Can you work these out from the model? Positions are in its coordinate system, mm. A direction names the side the tool comes from. Give positions to 0.01 mm unless a question says otherwise; leave off trailing zeros. Loops run counter-clockwise (first coordinate to the right, second up) from the corner with the lowest first, then second, coordinate; pieces in that order, holes last. Notation, with made-up numbers: M 72.25,69 L 92.25,69 A23 cw 92.25,91 Z; hole C -3.75,-29.5 d2. An arc over 180 degrees is marked long. Put each result on its own line as item: value. Start each with the question number.
1) Imagine slicing it at C-C (z = -20). Write out the boundary of the cut face in (x, y).
2) If we mould it in two halves opening along X, with no side actions, what happens to faces 1 (the flat face through (35, 0, -15)), 2 (the cylindrical face through (0.676, 0.088, -27.854)), 3 (the flat face through (30, 1, 0)), 4 (the cylindrical face through (-26.241, 2.685, 2.465))? For each: +X half, -X half, draft (parallel to the pull), parting line (faces both ways), or undercut.
3) Imagine slicing it at D-D (y = 3.5). Write out the boundary of the cut face in (x, z), then the cut area to 3 significant figures.
4) Please list where these lines run through material, in increasing order: line 1 along Z through (x, y) = (23.75, 1.5); line 2 along X through (y, z) = (-1.75, -25); line 3 along X through (y, z) = (-0.75, -18). Write a range as from..to.
5) Imagine slicing it at A-A (x = 23.75). Write out the boundary of the cut face in (y, z), then the cut area to 3 significant figures.
6) For P1, Ø6, axis at x = 23.75, z = -5.76, coming from the +Y side, with a flat end and sliding along its axis, tell me the tip position at first contact or that it passes through.
7) For faces 5 (the cylindrical face through (-26.241, 2.685, -32.535)), 6 (the cylindrical face through (-25.987, 1.476, -25.618)), which set-ups out of +Z, -Z, +X, -X, +Y, -Y let a thin tool reach every point of the face, with its end or its side?
8) Imagine slicing it at B-B (y = -3.75). State how many separate pieces and enclosed holes the cut face has, then the cut area to 3 significant figures.
from build123d import *

# Parameters (mm, degrees)
SKETCH1_W                = 70
SKETCH1_H                = 12.5
BOSS_EXTRUDE1_DEPTH      = 30
BOSS_EXTRUDE3_DEPTH      = 5
BOSS_EXTRUDE3_DEPTH_BACK = 35
CUT_EXTRUDE1_START       = -66
CUT_EXTRUDE1_DEPTH       = 66
SKETCH7_R                = 2.25
CUT_EXTRUDE2_DEPTH       = 66


with BuildPart() as part:
    # Sketch1 → Boss-Extrude1 (new body)
    with BuildSketch(Plane.XY):
        Rectangle(SKETCH1_W, SKETCH1_H)
    extrude(amount=-BOSS_EXTRUDE1_DEPTH)

    # Sketch2 → Boss-Extrude3 (add, two sides: drawn at the far end of the back side and taken through both)
    with BuildSketch(Plane.XY.offset(-BOSS_EXTRUDE3_DEPTH_BACK)):
        with BuildLine():
            Line((-10, -6.25), (10, -6.25))
            ThreePointArc((10, -6.25), (17.5, 1.25), (25, -6.25))
            Line((25, -6.25), (30, -6.25))
            ThreePointArc((30, -6.25), (26.338834765, 2.588834765), (17.5, 6.25))
            Line((17.5, 6.25), (-17.5, 6.25))
            ThreePointArc((-17.5, 6.25), (-26.338834765, 2.588834765), (-30, -6.25))
            Line((-30, -6.25), (-25, -6.25))
            ThreePointArc((-25, -6.25), (-17.5, 1.25), (-10, -6.25))
        make_face()
    extrude(amount=BOSS_EXTRUDE3_DEPTH + BOSS_EXTRUDE3_DEPTH_BACK)

    # Sketch5 → Cut-Extrude1 (cut)
    with BuildSketch(Plane.XY.offset(5).offset(CUT_EXTRUDE1_START)):
        with BuildLine():
            Line((-25, -6.25), (-10, -6.25))
            ThreePointArc((-10, -6.25), (-17.5, 1.25), (-25, -6.25))
        make_face()
        with BuildLine():
            Line((10, -6.25), (25, -6.25))
            ThreePointArc((25, -6.25), (17.5, 1.25), (10, -6.25))
        make_face()
    extrude(amount=CUT_EXTRUDE1_DEPTH, mode=Mode.SUBTRACT)

    # Sketch7 → Cut-Extrude2 (cut)
    with BuildSketch(Plane(origin=(0, 6.25, 0), x_dir=(1, 0, 0), z_dir=(0, 1, 0))):
        with Locations(Location((0, 0, 0), (0, 0, 270))):
            Circle(SKETCH7_R)
        with Locations(Location((0, 30, 0), (0, 0, 270))):
            Circle(SKETCH7_R)
        with Locations(Location((23.75, 25.372099054, 0), (0, 0, 270))):
            Circle(SKETCH7_R)
        with Locations(Location((23.75, 5.759402661, 0), (0, 0, 270))):
            Circle(SKETCH7_R)
        with Locations(Location((-23.75, 25.372099054, 0), (0, 0, 236.251011404))):
            Circle(SKETCH7_R)
        with Locations(Location((-23.75, 5.759402661, 0), (0, 0, 236.251011404))):
            Circle(SKETCH7_R)
    extrude(amount=-CUT_EXTRUDE2_DEPTH, mode=Mode.SUBTRACT)


solid = part.part
Recorded:
1. outline: M -35,-6.25 L -25,-6.25 A7.5 cw -10,-6.25 L 10,-6.25 A7.5 cw 25,-6.25 L 35,-6.25 L 35,6.25 L -35,6.25 Z
2. face 1: +X half
2. face 2: undercut
2. face 3: draft
2. face 4: -X half
3. outline: M -35,-30 L -25.32,-30 L -25.32,-35 L 25.32,-35 L 25.32,-30 L 35,-30 L 35,0 L 25.32,0 L 25.32,5 L -25.32,5 L -25.32,0 L -35,0 Z; hole C -23.75,-25.37 d4.5; hole C -23.75,-5.76 d4.5; hole C 0,-30 d4.5; hole C 0,0 d4.5; hole C 23.75,-25.37 d4.5; hole C 23.75,-5.76 d4.5
3. area: 2,510 mm²
4. line 1: -35..-27.62, -23.12..-8.01, -3.51..5
4. line 2: -35..-25.97, -11.5..11.5, 25.97..35
4. line 3: -35..-22.6, -12.4..12.4, 22.6..35
5. outline: M -2.1,-35 L 4.58,-35 L 4.58,-30 L 6.25,-30 L 6.25,-27.62 L -2.1,-27.62 Z; M -2.1,-23.12 L 6.25,-23.12 L 6.25,-8.01 L -2.1,-8.01 Z; M -2.1,-3.51 L 6.25,-3.51 L 6.25,0 L 4.58,0 L 4.58,5 L -2.1,5 Z
5. area: 242 mm²
6. P1: y = 6.25
7. face 5: -Z, -X, +Y
7. face 6: +Y, -Y
8. separate pieces: 3
8. enclosed holes: 2
8. area: 1,510 mm²
